The drawing under review shows one solid part. Ordinate dimensions are in mm from its lowest x, y, z. A direction names the side the tool comes from. Round coordinates to 2 decimals unless told otherwise and drop trailing zeros. Order: outer loops, then holes, each group sorted by start corner. A loop starts at its lowest first (then second) coordinate and runs counter-clockwise, first axis right, second up. Notation, with made-up numbers: M 7.5,24.5 L 49.5,24.5 A17 cw 49.5,40.5 Z; hole C 37,37 d4. An arc over 180 degrees is marked long. Answer as a JSON object with one key per item and string values. Group by question number.
1. Add section B-B on x = 13.5. State the section outline as (y, z) points, and give its area (3 significant figures).
2. To check wall thickness, follow probe 1 along Y at (x, z) = (21.75, 3); probe 2 along X at (y, z) = (0.9, 8); probe 3 along Z at (x, y) = (7.5, 1.7). State the ranges of each line that lie inside material, in increasing order. Write a range as [from, to].
3. Add section D-D on z = 13.5. State the section outline as (x, y) points, and give its area (3 significant figures).
4. Add section C-C on y = 0.4. State the section outline as (x, z) points, and give its area (3 significant figures).
5. Machinability: for the marked faces 1 and 2, which of the approach directions +Z, -Z, +X, -X, +Y, -Y give a long, thin tool a straight path to every point of the face, cutting with its end or side? Answer none if there is none.
6. Add section A-A on z = 1.5. State the section outline as (x, y) points.
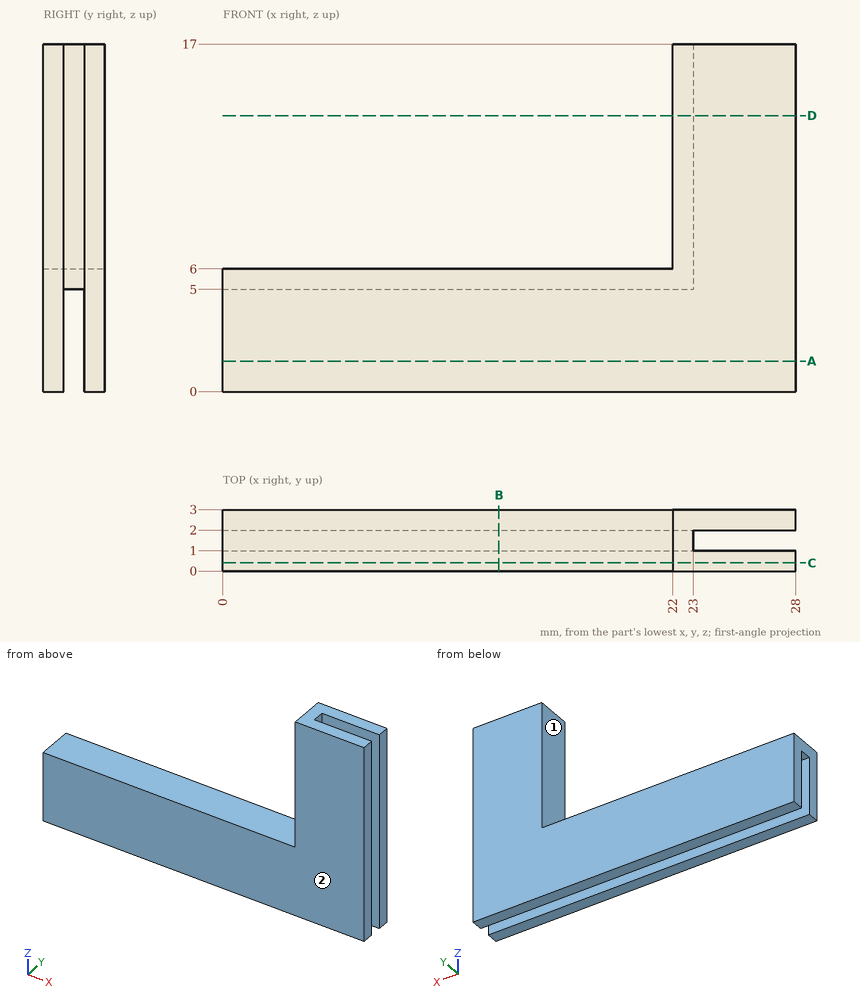
Recorded:
{
 "1": {"outline": "M 0,0 L 1,0 L 1,5 L 2,5 L 2,0 L 3,0 L 3,6 L 0,6 Z", "area": "13.0 mm²"},
 "2": {"probe 1": "y = [0, 1], [2, 3]", "probe 2": "x = [22, 28]", "probe 3": "z = [5, 6]"},
 "3": {"outline": "M 22,0 L 28,0 L 28,1 L 23,1 L 23,2 L 28,2 L 28,3 L 22,3 Z", "area": "13.0 mm²"},
 "4": {"outline": "M 0,0 L 28,0 L 28,17 L 22,17 L 22,6 L 0,6 Z", "area": "234 mm²"},
 "5": {"face 1": "+Z, -X, +Y, -Y", "face 2": "+Z, -Z, +X, -X, -Y"},
 "6": {"outline": "M 0,0 L 28,0 L 28,1 L 0,1 Z; M 0,2 L 28,2 L 28,3 L 0,3 Z"}
}
